Geometry: final body of the model. Coordinates: model frame, mm. Face numbers are marked on the shaded views. Round coordinates to 2 decimals unless told otherwise and drop trailing zeros. Loops run counter-clockwise (first coordinate to the right, second up) from the corner with the lowest first, then second, coordinate; pieces in that order, holes last. Notation, with made-up numbers: (72, -31) - (78, -31) arc R9 ccw to (78, -20) - close; hole circle Ø3 at (-24.5, -2). An arc over 180 degrees is marked (long way). Return JSON: item names as keys, results as strings. Group by question number.
1. Section A-A on y = 4.75. Return loops of the section in (x, z).
2. First-contact query: pin 1 Ø5 at (x, z) = (5.5, 2.5) entering from +Y; pin 2 Ø4 at (x, z) = (0.5, 1.5) entering from -Y; pin 3 Ø2 at (x, z) = (5, -5.5) entering from +Y. Flat tips, straight axial feed; report the tip coordinate or a pass-through.
3. Section B-B on y = 7.25. Return loops of the section in (x, z).
4. Draft query along X for the marked faces 1, 2 and 3. Return one class per face: +X half, -X half, draft (parallel to the pull), parting line (faces both ways), or undercut.
5. Material intervals for probe 1 along Y at (x, z) = (2.25, 0.75); probe 2 along X at (y, z) = (3.25, -1.25); probe 3 along Z at (x, y) = (0, 4), sorted ascending.
6. Section C-C on y = 9.25. Return loops of the section in (x, z).
from build123d import *

# Parameters (mm, degrees)
BOSS_EXTRUDE1_DEPTH = 10
FILLET1_R           = 4
SKETCH2_R           = 4.1
CUT_EXTRUDE1_DEPTH  = 8


with BuildPart() as part:
    # Sketch1 → Boss-Extrude1 (new body)
    with BuildSketch(Plane(origin=(0, 0, 0), x_dir=(1, 0, 0), z_dir=(0, 1, 0))):
        Polygon((-6.812793916, 3.588291941), (-6.513948935, -4.105906632), (0.298844981, -7.694198573), (6.812793916, -3.588291941), (6.513948935, 4.105906632), (-0.298844981, 7.694198573), align=None)
    extrude(amount=BOSS_EXTRUDE1_DEPTH)

    # Fillet1
    fillet1_edges = [part.edges().sort_by_distance(p)[0] for p in [
        (-3.107551977, 10, 5.900052602),
        (3.555819448, 10, 5.641245257),
        (6.663371426, 10, -0.258807345),
        (3.107551977, 10, -5.900052602),
        (-3.555819448, 10, -5.641245257),
        (-6.663371426, 10, 0.258807345),
    ]]
    fillet(fillet1_edges, radius=FILLET1_R)

    # Sketch2 → Cut-Extrude1 (cut)
    with BuildSketch(Plane.XZ):
        Circle(SKETCH2_R)
    extrude(amount=-CUT_EXTRUDE1_DEPTH, mode=Mode.SUBTRACT)


solid = part.part
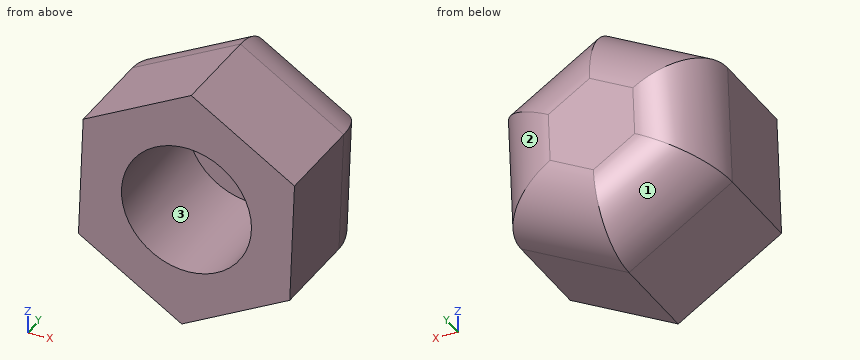
Taken from the geometry:
{
 "1": {"outline": "(-6.81, -3.59) - (-0.3, -7.69) - (6.51, -4.11) - (6.81, 3.59) - (0.3, 7.69) - (-6.51, 4.11) - close; hole circle Ø8.2 at (0, 0)"},
 "2": {"pin 1": "y = 9.98", "pin 2": "y = 8", "pin 3": "y = 7.89"},
 "3": {"outline": "(-6.61, -3.48) - (-0.29, -7.46) - (6.32, -3.98) - (6.61, 3.48) - (0.29, 7.46) - (-6.32, 3.98) - close; hole circle Ø8.2 at (0, 0)"},
 "4": {"face 1": "-X half", "face 2": "+X half", "face 3": "undercut"},
 "5": {"probe 1": "8 to 10", "probe 2": "-6.72 to -3.9, 3.9 to 6.62", "probe 3": "-7.54 to -4.1, 4.1 to 7.54"},
 "6": {"outline": "(-5.11, -2.69) - (-0.22, -5.77) - (4.88, -3.08) - (5.11, 2.69) - (0.22, 5.77) - (-4.88, 3.08) - close"}
}
